Verification items for the finished model (mm, model axes). Give positions to 0.01 mm unless a question says otherwise; leave off trailing zeros.
(1) Gauge pin test, flat end, axial feed: pin 1 (3 mm diameter, centred on y = 18.5, z = 1226.5, fed in from -X). Record the tip position at first contact, or that the pin passes through.
(2) Scan lines: L1, parallel to X at y = 4, z = 1114.5; L2, parallel to X at y = 13, z = 1883; L3, parallel to Y at x = 6.5, z = 232.5. Record each from-to range of solid material in increasing order.
(3) Sectioned sample at A-A on z = 159.5. Count the separate pieces of the cut face and the enclosed holes in it, plus the area to 3 significant figures.
```python
from build123d import *

# Parameters (mm, degrees)
CROQUIS1_W              = 5.700927171
CROQUIS1_H              = 5.669703343
CROQUIS1_W_2            = 5.669703343
CROQUIS1_H_2            = 5.700927171
SALIENTE_EXTRUIR1_DEPTH = 2000


with BuildPart() as part:
    # Croquis1 → Saliente-Extruir1 (new body)
    with BuildSketch(Plane.XY):
        with BuildLine():
            Line((16, 0), (16, 3.526999273))
            Line((16, 3.526999273), (13.842037149, 3.526999273))
            Line((13.842037149, 3.526999273), (13.842037149, 1.764099906))
            ThreePointArc((13.842037149, 1.764099906), (11.014894419, 3.909691284), (10.589261103, 7.433202979))
            ThreePointArc((10.589261103, 7.433202979), (12.773071968, 10.642430452), (16, 12.8))
            Line((16, 12.8), (20, 12.8))
            Line((20, 12.8), (24, 12.8))
            ThreePointArc((24, 12.8), (27.226928032, 10.642430452), (29.410738897, 7.433202979))
            ThreePointArc((29.410738897, 7.433202979), (28.985105581, 3.909691284), (26.157962851, 1.764099906))
            Line((26.157962851, 1.764099906), (26.157962851, 3.526999273))
            Line((26.157962851, 3.526999273), (24, 3.526999273))
            Line((24, 3.526999273), (24, 0))
            Line((24, 0), (40, 0))
            Line((40, 0), (40, 16))
            Line((40, 16), (36.473000727, 16))
            Line((36.473000727, 16), (36.473000727, 13.842037149))
            Line((36.473000727, 13.842037149), (38.235900094, 13.842037149))
            ThreePointArc((38.235900094, 13.842037149), (36.090308716, 11.014894419), (32.566797021, 10.589261103))
            ThreePointArc((32.566797021, 10.589261103), (29.357569548, 12.773071968), (27.2, 16))
            Line((27.2, 16), (27.2, 20))
            Line((27.2, 20), (27.2, 24))
            ThreePointArc((27.2, 24), (29.357569548, 27.226928032), (32.566797021, 29.410738897))
            ThreePointArc((32.566797021, 29.410738897), (36.090308716, 28.985105581), (38.235900094, 26.157962851))
            Line((38.235900094, 26.157962851), (36.473000727, 26.157962851))
            Line((36.473000727, 26.157962851), (36.473000727, 24))
            Line((36.473000727, 24), (40, 24))
            Line((40, 24), (40, 40))
            Line((40, 40), (24, 40))
            Line((24, 40), (24, 36.473000727))
            Line((24, 36.473000727), (26.157962851, 36.473000727))
            Line((26.157962851, 36.473000727), (26.157962851, 38.235900094))
            ThreePointArc((26.157962851, 38.235900094), (28.985105581, 36.090308716), (29.410738897, 32.566797021))
            ThreePointArc((29.410738897, 32.566797021), (27.226928032, 29.357569548), (24, 27.2))
            Line((24, 27.2), (20, 27.2))
            Line((20, 27.2), (16, 27.2))
            ThreePointArc((16, 27.2), (12.773071968, 29.357569548), (10.589261103, 32.566797021))
            ThreePointArc((10.589261103, 32.566797021), (11.014894419, 36.090308716), (13.842037149, 38.235900094))
            Line((13.842037149, 38.235900094), (13.842037149, 36.473000727))
            Line((13.842037149, 36.473000727), (16, 36.473000727))
            Line((16, 36.473000727), (16, 40))
            Line((16, 40), (0, 40))
            Line((0, 40), (0, 24))
            Line((0, 24), (3.526999273, 24))
            Line((3.526999273, 24), (3.526999273, 26.157962851))
            Line((3.526999273, 26.157962851), (1.764099906, 26.157962851))
            ThreePointArc((1.764099906, 26.157962851), (3.909691284, 28.985105581), (7.433202979, 29.410738897))
            ThreePointArc((7.433202979, 29.410738897), (10.642430452, 27.226928032), (12.8, 24))
            Line((12.8, 24), (12.8, 20))
            Line((12.8, 20), (12.8, 16))
            ThreePointArc((12.8, 16), (10.642430452, 12.773071968), (7.433202979, 10.589261103))
            ThreePointArc((7.433202979, 10.589261103), (3.909691284, 11.014894419), (1.764099906, 13.842037149))
            Line((1.764099906, 13.842037149), (3.526999273, 13.842037149))
            Line((3.526999273, 13.842037149), (3.526999273, 16))
            Line((3.526999273, 16), (0, 16))
            Line((0, 16), (0, 0))
            Line((0, 0), (16, 0))
        make_face()
        with Locations((4.415111636, 4.598351308)):
            Rectangle(CROQUIS1_W, CROQUIS1_H, mode=Mode.SUBTRACT)
        with Locations((4.598351308, 35.584888365)):
            Rectangle(CROQUIS1_W_2, CROQUIS1_H_2, mode=Mode.SUBTRACT)
        with Locations((35.584888365, 35.401648693)):
            Rectangle(CROQUIS1_W, CROQUIS1_H, mode=Mode.SUBTRACT)
        with Locations((35.401648693, 4.415111636)):
            Rectangle(CROQUIS1_W_2, CROQUIS1_H_2, mode=Mode.SUBTRACT)
        with BuildLine():
            ThreePointArc((16.6, 20), (17.595836944, 17.595836944), (20, 16.6))
            ThreePointArc((20, 16.6), (22.404163056, 17.595836944), (23.4, 20))
            ThreePointArc((23.4, 20), (22.404163056, 22.404163056), (20, 23.4))
            ThreePointArc((20, 23.4), (17.595836944, 22.404163056), (16.6, 20))
        make_face(mode=Mode.SUBTRACT)
    extrude(amount=SALIENTE_EXTRUIR1_DEPTH)


solid = part.part
```
Ans:
1. pin 1: stops at x = 12.8
2. L1: x = 0 to 1.56, 7.27 to 10.96, 29.04 to 32.57, 38.24 to 40
2. L2: x = 0 to 2.07, 10.86 to 29.14, 37.93 to 40
2. L3: y = 0 to 1.76, 7.43 to 10.42, 29.58 to 32.73, 38.44 to 40
3. separate pieces: 1
3. enclosed holes: 5
3. area: 687 mm2
